The listing builds one solid part. Answer for the finished solid, in the listing's coordinates (mm). Face numbers are marked on the shaded views. A direction names the side the tool comes from. Round coordinates to 2 decimals unless told otherwise and drop trailing zeros. Order: outer loops, then holes, each group sorted by start corner. A loop starts at its lowest first (then second) coordinate and runs counter-clockwise, first axis right, second up. Notation, with made-up numbers: M -22,11 L -13,11 A22 ccw -13,35 Z; hole C 79,57 d2. An arc over 180 degrees is marked long. Put each result on its own line as item: value. Start each with the question number.
1. The mould has two halves that part along Z. Classify the marked faces 4, 5 and 6: +Z half, -Z half, draft (parallel to the pull), parting line (faces both ways), or undercut.
2. Consider line 1 (X direction, y = 1.5, z = -3); line 2 (Z direction, x = 3, y = -1.5); line 3 (Z direction, x = -3.5, y = -2.5). Determine where each line is inside the solid, lowest interval first.
3. Which of the six approach directions +Z, -Z, +X, -X, +Y, -Y give full straight-line access (tool end or side, diameter ignored) to the marked faces 1, 2 and 3?
4. The part is cut by section A-A (x = 3). Give the vertices of the cut face in (y, z), then the cut area to 3 significant figures.
5. The part is cut by section B-B (x = -0.75). Give the vertices of the cut face in (y, z).
6. Each of these flat-tipped pins is pushed along its axis until it touches: pin 1 Ø1.1 at (y, z) = (-0.5, 1.5) entering from -X; pin 2 Ø1.5 at (x, z) = (-2.5, 2.5) entering from +Y; pin 3 Ø0.5 at (y, z) = (1, -1.5) entering from -X; pin 4 Ø3 at (x, y) = (3.5, -3) entering from -Z. Where does it stop, or does it pass through?
from build123d import *

# Parameters (mm, degrees)
CHAMFER1_SIZE      = 0.5
CUT_EXTRUDE1_DEPTH = 2.5


with BuildPart() as part:
    # Sketch1 → Revolve1 (revolve)
    with BuildSketch(Plane.XY):
        Polygon((-5, 0), (-5, 3.75), (-4.5, 4.25), (0, 4.25), (0, 2.5), (12, 2.5), (12, 0), align=None)
    revolve(axis=Axis((12, 0, 0), (-1, 0, 0)))

    # Chamfer1
    chamfer1_edges = [part.edges().sort_by_distance(p)[0] for p in [
        (12, -2.5, 0),
    ]]
    chamfer(chamfer1_edges, length=CHAMFER1_SIZE)

    # Sketch2 → Cut-Revolve1 (revolve, cut)
    with BuildSketch(Plane.XY):
        Polygon((-5, 0), (-5, 2), (-2.5, 2), (-1.964101615, 0), align=None)
    revolve(axis=Axis((-1.964101615, 0, 0), (-1, 0, 0)), mode=Mode.SUBTRACT)

    # Sketch3 → Cut-Extrude1 (cut)
    with BuildSketch(Plane(origin=(-5, 0, 0), x_dir=(0, 0, -1), z_dir=(1, 0, 0))):
        Polygon((-2, 1.154700538), (-2, -1.154700538), (0, -2.309401077), (2, -1.154700538), (2, 1.154700538), (0, 2.309401077), align=None)
    extrude(amount=CUT_EXTRUDE1_DEPTH, mode=Mode.SUBTRACT)


solid = part.part
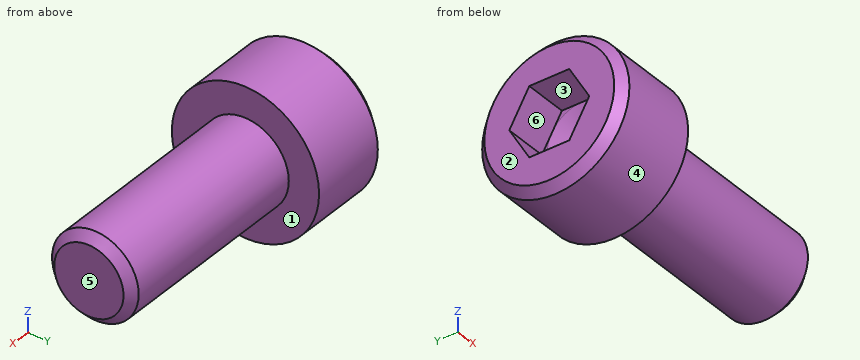
Resolved:
1. face 4: parting line
1. face 5: draft
1. face 6: undercut
2. line 1: -5 to 0
2. line 2: -2 to 2
2. line 3: -3.44 to 3.44
3. face 1: +X
3. face 2: +Z, -Z, -X, +Y, -Y
3. face 3: -X
4. outline: C 0,0 d5
4. area: 19.6 mm2
5. outline: C 0,0 d8.5
6. pin 1: x = -5
6. pin 2: y = 3.87
6. pin 3: x = -2.5
6. pin 4: z = -2
